Check sheet for the modelled part. Datum: model origin and axes. Units: mm. A direction names the side the tool comes from. Round coordinates to 2 decimals unless told otherwise and drop trailing zeros. Write each loop counter-clockwise with the first axis right and the second up, starting at its lowest first coordinate (ties: lowest second). Pieces come first, ordered by that corner, then holes. Notation, with made-up numbers: (33, 83.5) -> (79, 83.5) arc R33 ccw to (79, 111.5) -> close; hole circle Ø1 at (-7, 62.25). An arc over 180 degrees is marked (long way). One line per item, written item: value.
from build123d import *

# Parameters (mm, degrees)
BOSS_EXTRUDE1_DEPTH = 5
SKETCH1_13_R        = 1.1
CUT_EXTRUDE2_DEPTH  = 10
FILLET1_R           = 2
BOSS_EXTRUDE2_DEPTH = 11


with BuildPart() as part:
    # Sketch1 → Boss-Extrude1 (new body)
    with BuildSketch(Plane.XY):
        with BuildLine():
            Line((27.361611466, 75.175409663), (32.833933759, 90.210491595))
            ThreePointArc((32.833933759, 90.210491595), (9.201192242, 95.558035043), (-15.017708644, 94.818080697))
            Line((-15.017708644, 94.818080697), (-12.514757203, 79.015067248))
            ThreePointArc((-12.514757203, 79.015067248), (7.667660202, 79.631695869), (27.361611466, 75.175409663))
        make_face()
    extrude(amount=BOSS_EXTRUDE1_DEPTH)

    # Sketch1<13> → Cut-Extrude2 (cut)
    with BuildSketch(Plane.XY):
        with BuildLine():
            ThreePointArc((13.453363993, 84.941197291), (19.959187303, 83.651843029), (26.346302102, 81.864964213))
            Line((26.346302102, 81.864964213), (27.571711502, 85.672636967))
            ThreePointArc((27.571711502, 85.672636967), (20.887521597, 87.542626426), (14.079101854, 88.891950654))
            Line((14.079101854, 88.891950654), (13.453363993, 84.941197291))
        make_face()
        with Locations((8, 88)):
            Circle(SKETCH1_13_R)
    extrude(amount=CUT_EXTRUDE2_DEPTH, mode=Mode.SUBTRACT)

    # Fillet1
    fillet1_edges = [part.edges().sort_by_distance(p)[0] for p in [
        (26.346302102, 81.864964213, 2.5),
        (27.571711502, 85.672636967, 2.5),
        (14.079101854, 88.891950654, 2.5),
        (13.453363993, 84.941197291, 2.5),
        (-12.514757203, 79.015067248, 2.5),
        (-15.017708644, 94.818080697, 2.5),
        (27.361611466, 75.175409663, 2.5),
        (32.833933759, 90.210491595, 2.5),
    ]]
    fillet(fillet1_edges, radius=FILLET1_R - 0.0001)  # a hair under: the kernel refuses the full size

    # Sketch1<14> → Boss-Extrude2 (add)
    with BuildSketch(Plane.XY):
        with BuildLine():
            ThreePointArc((-0.5, 92.19088917), (-8.226985142, 88), (-0.5, 83.80911083))
            Line((-0.5, 83.80911083), (-0.5, 92.19088917))
        make_face()
        with BuildLine():
            Line((-0.5, 92.19088917), (-0.5, 83.80911083))
            ThreePointArc((-0.5, 83.80911083), (1.168178433, 85.616192721), (1.773014858, 88))
            ThreePointArc((1.773014858, 88), (1.168178433, 90.383807279), (-0.5, 92.19088917))
        make_face()
    extrude(amount=BOSS_EXTRUDE2_DEPTH)


solid = part.part
Item 1: Sectioned sample at D-D on x = -2.5. Enter the section's corners in (y, z).
Answer:
outline: (79.96, 0) -> (95.97, 0) -> (95.97, 5) -> (92.95, 5) -> (92.95, 11) -> (83.05, 11) -> (83.05, 5) -> (79.96, 5) -> close
Item 2: Depth check by flat-ended pin: P1, Ø6, axis at y = 86, z = 7.5, coming from the -X side; P2, Ø1, axis at x = 27, y = 84, coming from the +Z side; P3, Ø6, axis at y = 79.5, z = 8.5, coming from the -X side; P4, Ø2, axis at y = 91, z = 9, coming from the -X side. Enter the tip coordinate at first touch or a pass-through.
Answer:
P1: stops at x = -13.88
P2: stops at z = 5
P3: passes through
P4: stops at x = -7.81
Item 3: Tool access check on faces 4 (the cylindrical face through (32.076, 89.839, 2.535)), 5 (the cylindrical face through (14.119, 85.407, 2.535)). Record the directions out of +Z, -Z, +X, -X, +Y, -Y that give a thin tool (end or side, any length) a straight path to the whole face; none if there is none.
Answer:
face 4: +Z, -Z, +X
face 5: +Z, -Z
Item 4: Sectioned sample at C-C on z = 9.25. Enter the section's corners in (x, y).
Answer:
outline: circle Ø10 at (-3.23, 88)
Item 5: Thickness scan on line 1 (Z direction, x = 27.5, y = 81); line 2 (Y direction, x = 16, z = 2.5); line 3 (Y direction, x = 8, z = 3). Record the ranges inside material, lowest first.
Answer:
line 1: z = 0 to 5
line 2: y = 78.38 to 84.5, 88.56 to 94.66
line 3: y = 79.6 to 86.9, 89.1 to 95.67
Item 6: Mould release check, pull along X, two halves, no side actions. Record for faces 1 (the flat face through (-13.776, 86.977, 2.465)), 2 (the cylindrical face through (8.59, 88.93, 2.46)), 3 (the cylindrical face through (27, 75.9, 2.5)): pulls with the +X half, pulls with the -X half, needs draft (parallel to the pull), parting line crosses it, or undercut.
Answer:
face 1: pulls with the -X half
face 2: undercut
face 3: parting line crosses it
Item 7: Sectioned sample at B-B on y = 91.75. Enter the section's corners in (x, z).
Answer:
outline: (-14.53, 0) -> (28.25, 0) -> (28.25, 5) -> (0.08, 5) -> (0.08, 11) -> (-6.53, 11) -> (-6.53, 5) -> (-14.53, 5) -> close
Item 8: Sectioned sample at A-A on x = 8. Enter the section's corners in (y, z), and give its area (3 significant figures).
Answer:
outline: (79.6, 0) -> (86.9, 0) -> (86.9, 5) -> (79.6, 5) -> close; (89.1, 0) -> (95.67, 0) -> (95.67, 5) -> (89.1, 5) -> close
area: 69.3 mm^2
